Source: CAD feature listing. Evaluate the final solid. Frame: model axes, mm. A direction names the side the tool comes from. Coordinates: 2 decimals unless noted, no trailing zeros. Loops run counter-clockwise (first coordinate to the right, second up) from the corner with the lowest first, then second, coordinate; pieces in that order, holes last.
```python
from build123d import *

# Parameters (mm, degrees)
SKETCH1_R                        = 37.5
BOSS_EXTRUDE1_DEPTH              = 10
SKETCH2_R                        = 32.5
BOSS_EXTRUDE2_DEPTH              = 11
SKETCH3_R                        = 19
BOSS_EXTRUDE3_DEPTH              = 12
SKETCH4_R                        = 32.5
BOSS_EXTRUDE4_DEPTH              = 12
BOSS_EXTRUDE5_DEPTH              = 15
FILLET1_R                        = 1
F_25_0MM_DOWEL_HOLE1_D           = 25
F_25_0MM_DOWEL_HOLE1_CSINK_D     = 25.05
F_25_0MM_DOWEL_HOLE1_CSINK_ANGLE = 90
SKETCH9_W                        = 15.8
SKETCH9_H                        = 44.975
CUT_EXTRUDE2_DEPTH               = 4.25
CUT_EXTRUDE3_DEPTH               = 4.25


with BuildPart() as part:
    # Sketch1 → Boss-Extrude1 (new body)
    with BuildSketch(Plane.XY):
        Circle(SKETCH1_R)
    extrude(amount=BOSS_EXTRUDE1_DEPTH)

    # Sketch2 → Boss-Extrude2 (add)
    with BuildSketch(Plane(origin=(0, 0, 0), x_dir=(-1, 0, 0), z_dir=(0, 0, -1))):
        Circle(SKETCH2_R)
    extrude(amount=BOSS_EXTRUDE2_DEPTH)

    # Sketch3 → Boss-Extrude3 (add)
    with BuildSketch(Plane(origin=(0, 0, -11), x_dir=(-1, 0, 0), z_dir=(0, 0, -1))):
        Circle(SKETCH3_R)
    extrude(amount=BOSS_EXTRUDE3_DEPTH)

    # Sketch4 → Boss-Extrude4 (add)
    with BuildSketch(Plane(origin=(0, 0, -23), x_dir=(-1, 0, 0), z_dir=(0, 0, -1))):
        Circle(SKETCH4_R)
    extrude(amount=BOSS_EXTRUDE4_DEPTH)

    # Sketch5 → Boss-Extrude5 (add)
    with BuildSketch(Plane.XY.offset(10)):
        with BuildLine():
            Line((0, 17.5), (0, 37.5))
            ThreePointArc((0, 37.5), (-18.75, 32.475952642), (-32.475952642, 18.75))
            Line((-32.475952642, 18.75), (-15.155444566, 8.75))
            ThreePointArc((-15.155444566, 8.75), (-8.75, 15.155444566), (0, 17.5))
        make_face()
        with BuildLine():
            Line((-15.155444566, -8.75), (-32.475952642, -18.75))
            ThreePointArc((-32.475952642, -18.75), (-18.75, -32.475952642), (0, -37.5))
            Line((0, -37.5), (0, -17.5))
            ThreePointArc((0, -17.5), (-8.75, -15.155444566), (-15.155444566, -8.75))
        make_face()
        with BuildLine():
            ThreePointArc((37.5, 0), (36.222218486, 9.705714191), (32.475952642, 18.75))
            Line((32.475952642, 18.75), (15.155444566, 8.75))
            ThreePointArc((15.155444566, 8.75), (16.90370196, 4.529333289), (17.5, 0))
            ThreePointArc((17.5, 0), (16.90370196, -4.529333289), (15.155444566, -8.75))
            Line((15.155444566, -8.75), (32.475952642, -18.75))
            ThreePointArc((32.475952642, -18.75), (36.222218486, -9.705714191), (37.5, 0))
        make_face()
    extrude(amount=BOSS_EXTRUDE5_DEPTH)

    # Fillet1
    # the kernel refuses this fillet: 1 mm, written as the material it takes off along each edge
    with BuildSketch(Plane(origin=(0, 0, 10), x_dir=(-0.8660254037844362, 0.5000000000000042, 0), z_dir=(0.5000000000000042, 0.8660254037844362, 0))) as fillet1_piece_1:
        with BuildLine():
            CenterArc((37.5 - FILLET1_R, -FILLET1_R), FILLET1_R, 0, 90)
            Line((37.5 - FILLET1_R, 0), (37.5, 0))
            Line((37.5, 0), (37.5, -FILLET1_R))
        make_face()
    revolve(axis=Axis((0, 0, 10), (0, 0, 1)), revolution_arc=60, mode=Mode.SUBTRACT)
    with BuildSketch(Plane(origin=(0, 0, 25), x_dir=(-0.9283987696572769, 0.37158542019144725, 0), z_dir=(-0.37158542019144725, -0.9283987696572769, 0))) as fillet1_piece_2:
        with BuildLine():
            CenterArc((17.5 + FILLET1_R, FILLET1_R), FILLET1_R, 180, 90)
            Line((17.5 + FILLET1_R, 0), (17.5, 0))
            Line((17.5, 0), (17.5, FILLET1_R))
        make_face()
    revolve(axis=Axis((0, 0, 25), (0, 0, -1)), revolution_arc=76.373144951, mode=Mode.SUBTRACT)
    with BuildSketch(Plane(origin=(0, 0, 25), x_dir=(0.06662916908749308, 0.9977778078443669, 0), z_dir=(0.9977778078443669, -0.06662916908749308, 0))) as fillet1_piece_3:
        with BuildLine():
            CenterArc((37.5 - FILLET1_R, -FILLET1_R), FILLET1_R, 0, 90)
            Line((37.5 - FILLET1_R, 0), (37.5, 0))
            Line((37.5, 0), (37.5, -FILLET1_R))
        make_face()
    revolve(axis=Axis((0, 0, 25), (0, 0, 1)), revolution_arc=67.640800977, mode=Mode.SUBTRACT)
    with BuildSketch(Plane(origin=(0, 0, 10), x_dir=(0, -1, 0), z_dir=(-1, 0, 0))) as fillet1_piece_4:
        with BuildLine():
            CenterArc((37.5 - FILLET1_R, -FILLET1_R), FILLET1_R, 0, 90)
            Line((37.5 - FILLET1_R, 0), (37.5, 0))
            Line((37.5, 0), (37.5, -FILLET1_R))
        make_face()
    revolve(axis=Axis((0, 0, 10), (0, 0, 1)), revolution_arc=60, mode=Mode.SUBTRACT)
    with BuildSketch(Plane(origin=(0, 0, 25), x_dir=(0.14239697126692002, -0.9898096294611445, 0), z_dir=(0.9898096294611445, 0.14239697126692002, 0))) as fillet1_piece_5:
        with BuildLine():
            CenterArc((17.5 + FILLET1_R, FILLET1_R), FILLET1_R, 180, 90)
            Line((17.5 + FILLET1_R, 0), (17.5, 0))
            Line((17.5, 0), (17.5, FILLET1_R))
        make_face()
    revolve(axis=Axis((0, 0, 25), (0, 0, -1)), revolution_arc=76.373144951, mode=Mode.SUBTRACT)
    with BuildSketch(Plane(origin=(0, 0, 25), x_dir=(-0.8974155134693206, -0.44118635085935703, 0), z_dir=(-0.44118635085935703, 0.8974155134693206, 0))) as fillet1_piece_6:
        with BuildLine():
            CenterArc((37.5 - FILLET1_R, -FILLET1_R), FILLET1_R, 0, 90)
            Line((37.5 - FILLET1_R, 0), (37.5, 0))
            Line((37.5, 0), (37.5, -FILLET1_R))
        make_face()
    revolve(axis=Axis((0, 0, 25), (0, 0, 1)), revolution_arc=67.640800977, mode=Mode.SUBTRACT)
    with BuildSketch(Plane(origin=(0, 0, 10), x_dir=(0.8660254037844433, 0.49999999999999195, 0), z_dir=(0.49999999999999195, -0.8660254037844433, 0))) as fillet1_piece_7:
        with BuildLine():
            CenterArc((37.5 - FILLET1_R, -FILLET1_R), FILLET1_R, 0, 90)
            Line((37.5 - FILLET1_R, 0), (37.5, 0))
            Line((37.5, 0), (37.5, -FILLET1_R))
        make_face()
    revolve(axis=Axis((0, 0, 10), (0, 0, 1)), revolution_arc=60, mode=Mode.SUBTRACT)
    with BuildSketch(Plane(origin=(0, 0, 25), x_dir=(0.7860017983903416, -0.6182242092697025, 0), z_dir=(-0.6182242092697025, -0.7860017983903416, 0))) as fillet1_piece_8:
        with BuildLine():
            CenterArc((17.5 + FILLET1_R, -FILLET1_R), FILLET1_R, 90, 90)
            Line((17.5, -FILLET1_R), (17.5, 0))
            Line((17.5, 0), (17.5 + FILLET1_R, 0))
        make_face()
    revolve(axis=Axis((0, 0, 25), (0, 0, 1)), revolution_arc=76.373144951, mode=Mode.SUBTRACT)
    with BuildSketch(Plane(origin=(0, 0, 25), x_dir=(0.8307863443818282, 0.5565914569849941, 0), z_dir=(-0.5565914569849941, 0.8307863443818282, 0))) as fillet1_piece_9:
        with BuildLine():
            CenterArc((37.5 - FILLET1_R, FILLET1_R), FILLET1_R, 270, 90)
            Line((37.5 - FILLET1_R, 0), (37.5, 0))
            Line((37.5, 0), (37.5, FILLET1_R))
        make_face()
    revolve(axis=Axis((0, 0, 25), (0, 0, -1)), revolution_arc=67.640800977, mode=Mode.SUBTRACT)

    # Ø25.0mm Dowel Hole1 (through all)
    with Locations(Plane.XY.offset(10)):
        with Locations((0, 0)):
            CounterSinkHole(F_25_0MM_DOWEL_HOLE1_D / 2, F_25_0MM_DOWEL_HOLE1_CSINK_D / 2, counter_sink_angle=F_25_0MM_DOWEL_HOLE1_CSINK_ANGLE)

    # Sketch9 → Cut-Extrude2 (cut, symmetric)
    with BuildSketch(Plane(origin=(0, 0, 0), x_dir=(1, 0, 0), z_dir=(0, 1, 0))):
        with Locations((7.9, 12.5125)):
            Rectangle(SKETCH9_W, SKETCH9_H)
    extrude(amount=CUT_EXTRUDE2_DEPTH, both=True, mode=Mode.SUBTRACT)

    # Sketch12 → Cut-Extrude3 (cut, symmetric)
    with BuildSketch(Plane(origin=(0, 0, 9.975), x_dir=(-1, 0, 0), z_dir=(0, 0, -1))):
        with BuildLine():
            Line((-11.755317946, 4.25), (-15.8, 4.25))
            Line((-15.8, 4.25), (-15.8, -4.25))
            Line((-15.8, -4.25), (-11.755317946, -4.25))
            ThreePointArc((-11.755317946, -4.25), (-12.5, 0), (-11.755317946, 4.25))
        make_face()
    extrude(amount=CUT_EXTRUDE3_DEPTH, both=True, mode=Mode.SUBTRACT)


solid = part.part
```
Q1. Material intervals for line 1 along Y through (x, z) = (0, -3); line 2 along Y through (x, z) = (0, -21); line 3 along Z through (x, y) = (23.5, 22), sorted ascending.
Q2. Section query B-B on z = -31. Return the cut outline in (x, y).
Q3. Reachability of faces 4 (the cylindrical face through (-8.767, -16.856, -16.916)), 5 (the flat face through (15.8, 0, -13)), 6 (the flat face through (-11, 31, 0)), 7 (the cylindrical face through (-8.86, 15.09, 16.9)) from +Z, -Z, +X, -X, +Y, -Y: full face, straight path, thin tool, end or side. Return the list, or none.
Q4. Draft query along Y for faces 1 (the cylindrical face through (-31, 9.76, -28.92)), 2 (the flat face through (-14, 0, -35)), 3 (the cylindrical face through (-8.64, -15.22, 16.9)). Return one class per face: released by +Y, released by -Y, zero draft, split by the parting line, or undercut.
Q5. Section query C-C on z = 2. Return the cut outline in (x, y), then the cut area to 3 significant figures.
Q6. Section query A-A on z = 19.5. Return the cut outline in (x, y), then the cut area to 3 significant figures.
Q7. First-contact query: pin 1 Ø5 at (y, z) = (18, 13.5) entering from -X; pin 2 Ø6 at (y, z) = (24, -1) entering from -X; pin 3 Ø4.5 at (x, z) = (13.5, -8) entering from +Y. Flat tips, straight axial feed; report the tip coordinate or a pass-through.
Resolved:
1. line 1: y = -32.5 to -12.5, 12.5 to 32.5
1. line 2: y = -19 to -12.5, 12.5 to 19
1. line 3: z = -35 to -23, -11 to 10
2. outline: circle Ø65 at (0, 0); hole (11.76, -4.25) - (15.8, -4.25) - (15.8, 4.25) - (11.76, 4.25) arc R12.5 ccw (long way) to start
3. face 4: none
3. face 5: +Z, -Z
3. face 6: -Z
3. face 7: +Z
4. face 1: split by the parting line
4. face 2: zero draft
4. face 3: undercut
5. outline: circle Ø75 at (0, 0); hole (11.76, -4.25) - (15.8, -4.25) - (15.8, 4.25) - (11.76, 4.25) arc R12.5 ccw (long way) to start
5. area: 3,900 mm2
6. outline: (-32.48, -18.75) arc R37.5 ccw to (0, -37.5) - (0, -17.5) arc R17.5 cw to (-15.16, -8.75) - close; (-32.48, 18.75) - (-15.16, 8.75) arc R17.5 cw to (0, 17.5) - (0, 37.5) arc R37.5 ccw to start; (15.16, -8.75) - (32.48, -18.75) arc R37.5 ccw to (32.48, 18.75) - (15.16, 8.75) arc R17.5 cw to start
6. area: 1,730 mm2
7. pin 1: stops at x = -32.48
7. pin 2: stops at x = -30.95
7. pin 3: stops at y = 30.49
